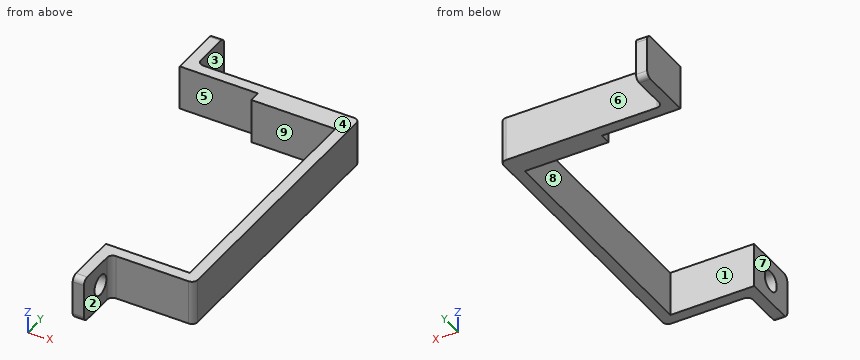
from build123d import *

# Parameters (mm, degrees)
F1_DEPTH = 8
F3_R     = 1.8
F2_R     = 1.8
F4_DEPTH = 25
F5_R     = 1
F6_R     = 1


with BuildPart() as f1:
    # F0 (on Top) → F1 (new body)
    with BuildSketch(Plane.XY):
        Polygon((3.5698827237, -0.7635216035), (-25.4301172763, -0.7635216035), (-25.4301172763, 7.2364783965), (-27.4301172763, 7.2364783965), (-27.4301172763, -2.7635216035), (-13.4301172763, -2.7635216035), (-13.4301172763, -4.7635216035), (1.5698827237, -4.7635216035), (1.5698827237, -48.7635216035), (-13.4301172763, -48.7635216035), (-13.4301172763, -58.7635216035), (-11.4301172763, -58.7635216035), (-11.4301172763, -50.7635216035), (3.5698827237, -50.7635216035), align=None)
    extrude(amount=F1_DEPTH)

    # F3 (on face) + F2 (on face) → F4 (cut)
    with BuildSketch(Plane(origin=(-13.4301172763, 0, 0), x_dir=(0, -1, 0), z_dir=(-1, 0, 0))):
        with Locations((53.7635216035, 4)):
            Circle(F3_R)
    with BuildSketch(Plane.YZ.offset(-25.4301172763)):
        with Locations((3.2364783965, 4)):
            Circle(F2_R)
    extrude(amount=-F4_DEPTH, dir=(-1, 0, 0), mode=Mode.SUBTRACT)

    # F5
    f5_edges = [f1.edges().sort_by_distance(p)[0] for p in [
        (-25.430117, -0.763522, 4),
        (-11.430117, -50.763522, 4),
        (3.569883, -50.763522, 4),
        (3.569883, -0.763522, 4),
    ]]
    fillet(f5_edges, radius=F5_R)

    # F6
    f6_edges = [f1.edges().sort_by_distance(p)[0] for p in [
        (-26.430117, 7.236478, 8),
        (-26.430117, 7.236478, 0),
        (-12.430117, -58.763522, 0),
        (-12.430117, -58.763522, 8),
    ]]
    fillet(f6_edges, radius=F6_R)


solid = f1.part
Read the model definition and answer for the solid it produces. Units are mm, in the model's axes. Face numbers are marked on the shaded views. A direction names the side the tool comes from. Coordinates: 2 decimals unless noted, no trailing zeros. Order: outer loops, then holes, each group sorted by start corner. A loop starts at its lowest first (then second) coordinate and runs counter-clockwise, first axis right, second up. Notation, with made-up numbers: (58.5, 20) -> (108.5, 20) arc R24 ccw to (108.5, 36) -> close; hole circle Ø8 at (42, 64.5). An arc over 180 degrees is marked (long way). Answer as a JSON object with one key per item and string values.
1) Each of these flat-tipped pins is pushed along its axis until it touches: pin 1 (2 mm diameter, centred on y = -53.76, z = 4, fed in from +X); pin 2 (2 mm diameter, centred on x = -1.5, z = 2, fed in from -Y); pin 3 (2 mm diameter, centred on y = -4, z = 4.5, fed in from -X); pin 4 (2 mm diameter, centred on y = -55, z = 2.5, fed in from +X). Where does it stop, or does it pass through?
Model answer:
{"pin 1": "passes through", "pin 2": "stops at y = -50.76", "pin 3": "stops at x = -13.43", "pin 4": "stops at x = -11.43"}
2) A cutting plane is placed at C-C, the plane x = -6. Determine the outline of the cut face in (y, z), plus the area to 3 significant figures.
Model answer:
{"outline": "(-50.76, 0) -> (-48.76, 0) -> (-48.76, 8) -> (-50.76, 8) -> close; (-4.76, 0) -> (-0.76, 0) -> (-0.76, 8) -> (-4.76, 8) -> close", "area": "48.0 mm²"}
3) Consider line 1 along Y through (x, z) = (1, 1); line 2 along Y through (x, z) = (-26, 6); line 3 along X through (y, z) = (-16, 7.75). Determine where each line is inside the solid, lowest interval first. Write a range as from..to.
Model answer:
{"line 1": "y = -50.76..-48.76, -4.76..-0.76", "line 2": "y = -2.76..7.24", "line 3": "x = 1.57..3.57"}
4) A cutting plane is placed at B-B, the plane z = 4. Determine the outline of the cut face in (x, y), plus the area to 3 significant figures.
Model answer:
{"outline": "(-27.43, -2.76) -> (-13.43, -2.76) -> (-13.43, -4.76) -> (1.57, -4.76) -> (1.57, -48.76) -> (-13.43, -48.76) -> (-13.43, -51.96) -> (-11.43, -51.96) -> (-11.43, -51.76) arc R1 cw to (-10.43, -50.76) -> (2.57, -50.76) arc R1 ccw to (3.57, -49.76) -> (3.57, -1.76) arc R1 ccw to (2.57, -0.76) -> (-24.43, -0.76) arc R1 cw to (-25.43, 0.24) -> (-25.43, 7.24) -> (-27.43, 7.24) -> close; (-13.43, -58.76) -> (-11.43, -58.76) -> (-11.43, -55.56) -> (-13.43, -55.56) -> close", "area": "243 mm²"}
5) The mould has two halves that part along Y. Classify the marked faces 6, 7, 8 and 9: released by +Y, released by -Y, zero draft, split by the parting line, or undercut.
Model answer:
{"face 6": "released by +Y", "face 7": "zero draft", "face 8": "undercut", "face 9": "undercut"}
6) A tool of negligible diameter and unlimited length cuts with its end or side. For the marked faces 1, 2, 3, 4 and 5, from which of +Z, -Z, +X, -X, +Y, -Y can it reach the whole face along a straight path? Write none if from no direction.
Model answer:
{"face 1": "+Z, -Z, -X", "face 2": "+Z, -Z, +X, -Y", "face 3": "+Z, -Z, +X, +Y", "face 4": "+Z, +X, -X, +Y, -Y", "face 5": "+Z, -Z, -X, -Y"}
7) A cutting plane is placed at A-A, the plane x = -12.5. Determine the outline of the cut face in (y, z), plus the area to 3 significant figures.
Model answer:
{"outline": "(-58.76, 1) arc R1 ccw to (-57.76, 0) -> (-48.76, 0) -> (-48.76, 8) -> (-57.76, 8) arc R1 ccw to (-58.76, 7) -> close; (-4.76, 0) -> (-0.76, 0) -> (-0.76, 8) -> (-4.76, 8) -> close; hole circle Ø3.6 at (-53.76, 4)", "area": "101 mm²"}
8) A cutting plane is placed at D-D, the plane y = -26. Determine the outline of the cut face in (x, z), plus the area to 3 significant figures.
Model answer:
{"outline": "(1.57, 0) -> (3.57, 0) -> (3.57, 8) -> (1.57, 8) -> close", "area": "16.0 mm²"}
